Input: dimensioned drawing with shaded views. Units: mm. Origin: part minimum x, y, z. Give positions to 0.01 mm unless a question says otherwise; leave off trailing zeros. Order: outer loops, then holes, each group sorted by start corner. A loop starts at its lowest first (then second) coordinate and runs counter-clockwise, first axis right, second up. Notation, with made-up numbers: (61.5, 26.5) -> (82.5, 26.5) arc R8 ccw to (82.5, 33.5) -> close; hole circle Ø4 at (-29, 73). An arc over 180 degrees is marked (long way). One line per question, with ' | ' between items. Start each with the question number.
(1) Section B-B (x = 250). Return loops of the section in (y, z).
(2) Ray query, L1, parallel to X at y = 240.5, z = 8.5; L2, parallel to X at y = 352.5, z = 3.5; L3, parallel to Y at x = 227, z = 13.5. Return the intervals inside material, ascending.
(3) First-contact query: pin 1 Ø8 at (x, z) = (388.5, 26.5) entering from -Y. Flat tip, straight axial feed; report the tip coordinate or a pass-through.
(4) Section C-C (y = 291). Return loops of the section in (x, z).
(5) Section A-A (z = 14). Return loops of the section in (x, y), then the cut area to 3 significant figures.
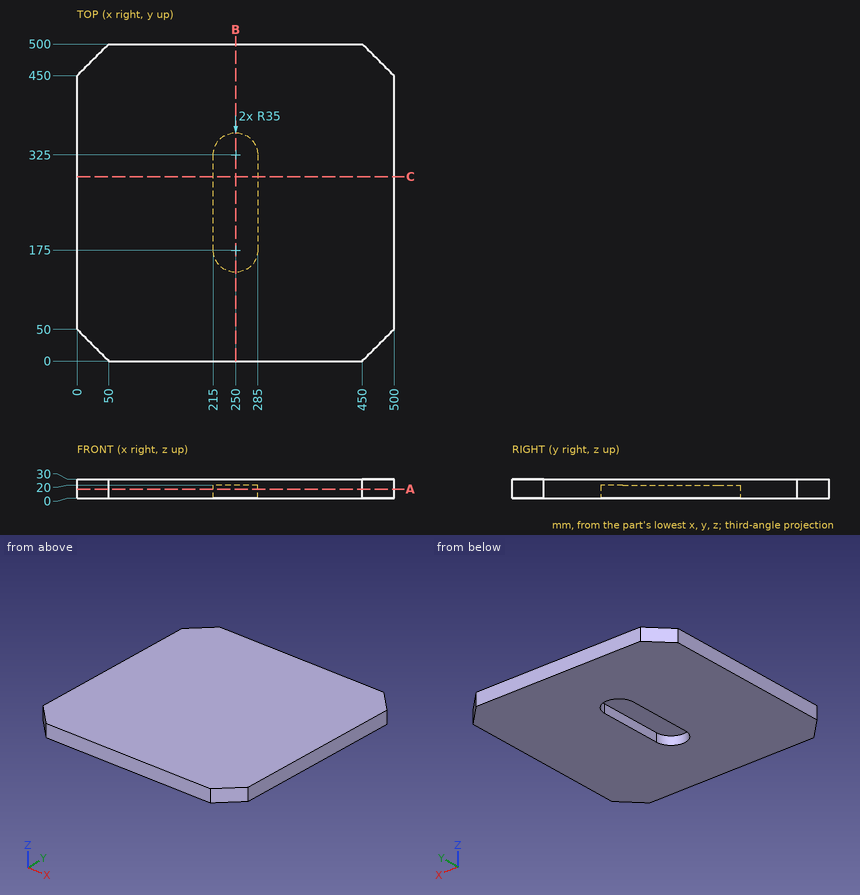
Response:
1) outline: (0, 0) -> (140, 0) -> (140, 20) -> (360, 20) -> (360, 0) -> (500, 0) -> (500, 30) -> (0, 30) -> close
2) L1: x = 0 to 215, 285 to 500 | L2: x = 0 to 228.35, 271.65 to 500 | L3: y = 0 to 148.62, 351.38 to 500
3) pin 1: stops at y = 0
4) outline: (0, 0) -> (215, 0) -> (215, 20) -> (285, 20) -> (285, 0) -> (500, 0) -> (500, 30) -> (0, 30) -> close
5) outline: (0, 50) -> (50, 0) -> (450, 0) -> (500, 50) -> (500, 450) -> (450, 500) -> (50, 500) -> (0, 450) -> close; hole (215, 175) arc R35 ccw to (285, 175) -> (285, 325) arc R35 ccw to (215, 325) -> close | area: 231,000 mm^2
